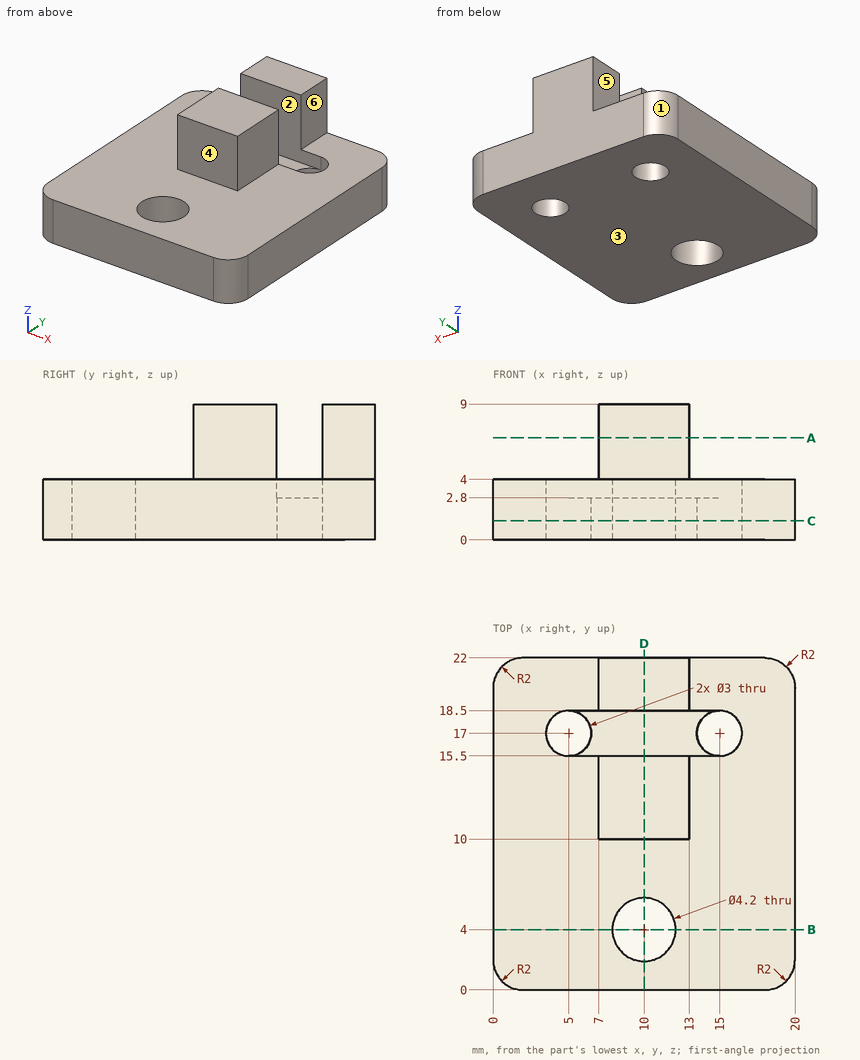
Check sheet for the drawn part. Datum: minimum x, y, z corner. Units: mm. A direction names the side the tool comes from. Give positions to 0.01 mm unless a question says otherwise; leave off trailing zeros. Loops run counter-clockwise (first coordinate to the right, second up) from the corner with the lowest first, then second, coordinate; pieces in that order, holes last.
1) Sectioned sample at B-B, the plane y = 4. Enter the section's corners in (x, z), then the cut area to 3 significant figures.
2) Sectioned sample at C-C, the plane z = 1.25. Enter the section's corners in (x, y).
3) Thickness scan on line 1 along X through (y, z) = (17, 1.7); line 2 along Y through (x, z) = (12.5, 5.25); line 3 along Y through (x, z) = (15, 2.65). Record the ranges inside material, lowest first.
4) Sectioned sample at A-A, the plane z = 6.75. Enter the section's corners in (x, y), then the cut area to 3 significant figures.
5) Set-up check for the marked faces 4, 5 and 6: record each of +Z, -Z, +X, -X, +Y, -Y from which the full face is reachable in a straight line by a thin tool's end or side.
6) Draft check along Y on the marked faces 1, 2 and 3. Enter one of: pulls with the +Y half, pulls with the -Y half, needs draft (parallel to the pull), parting line crosses it, or undercut.
7) Sectioned sample at D-D, the plane x = 10. Enter the section's corners in (y, z).
8) Depth check by flat-ended pin: pin 1 Ø12 at (x, y) = (12.5, 14) entering from -Z; pin 2 Ø4 at (x, y) = (3.5, 16.5) entering from +Z; pin 3 Ø1.5 at (y, z) = (11.5, 7) entering from +X; pin 4 Ø2.5 at (x, y) = (15, 17) entering from +Z. Enter the tip coordinate at first touch or a pass-through.
Answers:
1. outline: (0, 0) - (7.9, 0) - (7.9, 4) - (0, 4) - close; (12.1, 0) - (20, 0) - (20, 4) - (12.1, 4) - close
1. area: 63.2 mm2
2. outline: (0, 2) arc R2 ccw to (2, 0) - (18, 0) arc R2 ccw to (20, 2) - (20, 20) arc R2 ccw to (18, 22) - (2, 22) arc R2 ccw to (0, 20) - close; hole circle Ø3 at (5, 17); hole circle Ø4.2 at (10, 4); hole circle Ø3 at (15, 17)
3. line 1: x = 0 to 3.5, 6.5 to 13.5, 16.5 to 20
3. line 2: y = 10 to 15.5, 18.5 to 22
3. line 3: y = 0 to 15.5, 18.5 to 22
4. outline: (7, 10) - (13, 10) - (13, 15.5) - (7, 15.5) - close; (7, 18.5) - (13, 18.5) - (13, 22) - (7, 22) - close
4. area: 54.0 mm2
5. face 4: +Z, +X, -X, -Y
5. face 5: +Z, -X, +Y, -Y
5. face 6: +Z, +X, +Y, -Y
6. face 1: pulls with the +Y half
6. face 2: undercut
6. face 3: needs draft
7. outline: (0, 0) - (1.9, 0) - (1.9, 4) - (0, 4) - close; (6.1, 0) - (22, 0) - (22, 9) - (18.5, 9) - (18.5, 2.8) - (15.5, 2.8) - (15.5, 9) - (10, 9) - (10, 4) - (6.1, 4) - close
8. pin 1: stops at z = 0
8. pin 2: stops at z = 4
8. pin 3: stops at x = 13
8. pin 4: passes through
